Can you work these out from the model? Positions are in its coordinate system, mm. A direction names the side the tool comes from. Round coordinates to 2 decimals unless told otherwise and drop trailing zeros. Write each loop counter-clockwise with the first axis right and the second up, starting at its lowest first coordinate (ties: lowest second). Pieces come first, ordered by that corner, then holes.
Q1. If we section it at A-A (x = 8): Please give me the cut outline in (y, z).
Q2. If we section it at D-D (x = 94.5): Please give me the cut outline in (y, z).
Q3. If we section it at C-C (x = 46.5): Please give me the cut outline in (y, z), plus the area to 3 significant figures.
Q4. Please list where these lines run through material, in increasing order: line 1 along X through (y, z) = (33.5, 2.2); line 2 along Y through (x, z) = (63, 0.65); line 3 along X through (y, z) = (37, 2.55).
Q5. For faces 4 (the cylindrical face through (7.37, 22.17, 2.26)), 5 (the flat face through (25, 44, -2)), 6 (the flat face through (25, 25, 1)), which set-ups out of +Z, -Z, +X, -X, +Y, -Y let a thin tool reach every point of the face, with its end or its side?
Q6. I'm going to push flat-ended pins straight in: pin 1 Ø5 at (x, y) = (125.5, 10.5) entering from +Z; pin 2 Ø1.6 at (y, z) = (30.5, -1) entering from -X; pin 3 Ø2 at (y, z) = (32.5, -1.5) entering from +X. Where does each tip first touch, or does it pass through?
Q7. We'd pull the mould along Y, two halves only. Please class faces 1 (the flat face through (130, 43.1, 1)), 2 (the cylindrical face through (8.221, 26.686, 0.74)), 3 (the flat face through (76, 25, 0)): +Y half, -Y half, draft (parallel to the pull), parting line (faces both ways), or undercut.
Q8. If we section it at B-B (y = 13): Please give me the cut outline in (x, z), plus the area to 3 significant figures.
from build123d import *

# Parameters (mm, degrees)
PAD_DEPTH              = 3
SKETCH001_W            = 18.3
SKETCH001_H            = 18.1
POCKET_DEPTH           = 3.001
LINEARPATTERN_COUNT    = 4
LINEARPATTERN_PITCH    = 35
SKETCH002_W            = 129
SKETCH002_H            = 16
POCKET001_DEPTH        = 1.5
HOLE_D                 = 3.4
HOLE_CBORE_D           = 5.8
HOLE_CBORE_DEPTH       = 1.5
SKETCH004_W            = 22.3
SKETCH004_H            = 22.1
SKETCH004_W_2          = 18.3
SKETCH004_H_2          = 18.1
PAD001_DEPTH           = 2
LINEARPATTERN001_COUNT = 4
LINEARPATTERN001_PITCH = 35
FILLET_R               = 1
FILLET001_R            = 1
FILLET002_R            = 1


with BuildPart() as part:
    # Sketch → Pad (new body)
    with BuildSketch(Plane.XY):
        with BuildLine():
            Line((145, 49), (0, 49))
            Line((0, 49), (0, 0))
            Line((0, 0), (155, 0))
            Line((155, 0), (155, 39))
            ThreePointArc((155, 39), (152.071068, 46.071068), (145, 49))
        make_face()
    extrude(amount=PAD_DEPTH)

    # Sketch001 (on Face7 of Pad) → Pocket (cut, through all)
    with BuildSketch(Plane.XY.offset(3)):
        with Locations((25.15, 34.05)):
            Rectangle(SKETCH001_W, SKETCH001_H)
    pocket = extrude(amount=-POCKET_DEPTH, mode=Mode.SUBTRACT)

    # LinearPattern: Pocket ×4
    with Locations(*[(i * LINEARPATTERN_PITCH, 0, 0) for i in range(1, LINEARPATTERN_COUNT)]):
        add(pocket, mode=Mode.SUBTRACT)

    # Sketch002 (on Face5 of LinearPattern) → Pocket001 (cut)
    with BuildSketch(Plane.XY.offset(3)):
        with Locations((77.5, 11.5)):
            Rectangle(SKETCH002_W, SKETCH002_H)
    extrude(amount=-POCKET001_DEPTH, mode=Mode.SUBTRACT)

    # Hole (through all)
    with Locations(Plane.XY.offset(3)):
        with Locations((8, 25), (147, 25)):
            CounterBoreHole(HOLE_D / 2, HOLE_CBORE_D / 2, HOLE_CBORE_DEPTH)

    # Sketch004 (on Face4 of Hole) → Pad001 (join)
    with BuildSketch(Plane(origin=(0, 0, 0), x_dir=(1, 0, 0), z_dir=(0, 0, -1))):
        with Locations((25.15, -34.05)):
            Rectangle(SKETCH004_W, SKETCH004_H)
        with Locations((25.15, -34.05)):
            Rectangle(SKETCH004_W_2, SKETCH004_H_2, mode=Mode.SUBTRACT)
    pad001 = extrude(amount=PAD001_DEPTH)

    # LinearPattern001: Pad001 ×4
    with Locations(*[(i * LINEARPATTERN001_PITCH, 0, 0) for i in range(1, LINEARPATTERN001_COUNT)]):
        add(pad001)

    # Fillet
    fillet_edges = [part.edges().sort_by_distance(p)[0] for p in [
        (72.5, 49, 3),
    ]]
    fillet(fillet_edges, radius=FILLET_R)

    # Fillet001
    fillet001_edges = [part.edges().sort_by_distance(p)[0] for p in [
        (77, 0, 3),
    ]]
    fillet(fillet001_edges, radius=FILLET001_R)

    # Fillet002
    fillet002_edges = [part.edges().sort_by_distance(p)[0] for p in [
        (0, 24.5, 3),
    ]]
    fillet(fillet002_edges, radius=FILLET002_R)


solid = part.part
A:
1. outline: (0, 0) - (23.3, 0) - (23.3, 1.5) - (22.1, 1.5) - (22.1, 3) - (1, 3) arc R1 ccw to (0, 2) - close; (26.7, 0) - (49, 0) - (49, 2) arc R1 ccw to (48, 3) - (27.9, 3) - (27.9, 1.5) - (26.7, 1.5) - close
2. outline: (0, 0) - (23, 0) - (23, -2) - (25, -2) - (25, 3) - (19.5, 3) - (19.5, 1.5) - (3.5, 1.5) - (3.5, 3) - (1, 3) arc R1 ccw to (0, 2) - close; (43.1, -2) - (45.1, -2) - (45.1, 0) - (49, 0) - (49, 2) arc R1 ccw to (48, 3) - (43.1, 3) - close
3. outline: (0, 0) - (49, 0) - (49, 2) arc R1 ccw to (48, 3) - (19.5, 3) - (19.5, 1.5) - (3.5, 1.5) - (3.5, 3) - (1, 3) arc R1 ccw to (0, 2) - close
3. area: 123 mm2
4. line 1: x = 0.02 to 16, 34.3 to 51, 69.3 to 86, 104.3 to 121, 139.3 to 154.98
4. line 2: y = 0 to 25, 43.1 to 49
4. line 3: x = 0.16 to 16, 34.3 to 51, 69.3 to 86, 104.3 to 121, 139.3 to 154.84
5. face 4: +Z
5. face 5: -Z, +X, -X, +Y, -Y
5. face 6: +Z, -Z
6. pin 1: stops at z = 1.5
6. pin 2: stops at x = 14
6. pin 3: stops at x = 141.3
7. face 1: undercut
7. face 2: undercut
7. face 3: draft
8. outline: (0, 0) - (155, 0) - (155, 2) arc R1 ccw to (154, 3) - (142, 3) - (142, 1.5) - (13, 1.5) - (13, 3) - (1, 3) arc R1 ccw to (0, 2) - close
8. area: 271 mm2
